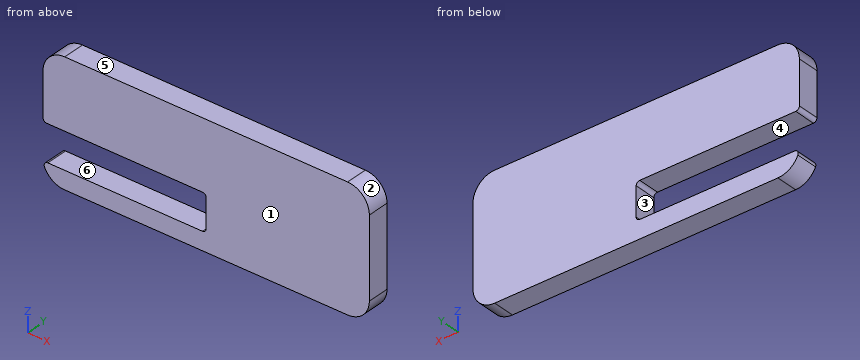
from build123d import *

# Parameters (mm, degrees)
CROQUIS1_W              = 45
CROQUIS1_H              = 17
SALIENTE_EXTRUIR1_DEPTH = 3
CROQUIS2_W              = 22.5
CROQUIS2_H              = 5
CORTAR_EXTRUIR1_DEPTH   = 3
REDONDEO1_R             = 3
REDONDEO4_R             = 0.5


with BuildPart() as part:
    # Croquis1 → Saliente-Extruir1 (new body)
    with BuildSketch(Plane(origin=(0, 0, 0), x_dir=(1, 0, 0), z_dir=(0, 1, 0))):
        with Locations((0, 1.429847209)):
            Rectangle(CROQUIS1_W, CROQUIS1_H)
    extrude(amount=SALIENTE_EXTRUIR1_DEPTH)

    # Croquis2 → Cortar-Extruir1 (cut)
    with BuildSketch(Plane(origin=(0, 3, 0), x_dir=(1, 0, 0), z_dir=(0, 1, 0))):
        with Locations((-11.25, 4.929847209)):
            Rectangle(CROQUIS2_W, CROQUIS2_H)
    extrude(amount=-CORTAR_EXTRUIR1_DEPTH, mode=Mode.SUBTRACT)

    # Redondeo1
    # the kernel refuses this fillet: 3 mm, written as the material it takes off along each edge
    with BuildSketch(Plane(origin=(-22.5, -7.395099729, -9.929847209), x_dir=(1, 0, 0), z_dir=(0, 1, 0))) as redondeo1_piece_1:
        with BuildLine():
            CenterArc((2.958039892, -3), REDONDEO1_R, 90, 80.405931773)
            Line((0, -2.5), (-0.059160798, -2.49))
            ThreePointArc((-0.059160798, -2.49), (-0.06, -1.25), (-0.06, 0))
            Line((-0.06, 0), (0, 0.06))
            Line((0, 0.06), (2.958039892, 0.06))
            Line((2.958039892, 0.06), (2.958039892, 0))
        make_face()
    extrude(amount=17.790199458, mode=Mode.SUBTRACT)
    with BuildSketch(Plane(origin=(22.5, -7.5, -9.929847209), x_dir=(-1, 0, 0), z_dir=(0, 1, 0)), Plane(origin=(22.5, -7.5, 7.070152791), x_dir=(0, 0, -1), z_dir=(0, 1, 0)), Plane(origin=(-22.5, -7.5, 7.070152791), x_dir=(1, 0, 0), z_dir=(0, 1, 0))) as redondeo1_piece_2:
        with BuildLine():
            CenterArc((REDONDEO1_R, REDONDEO1_R), REDONDEO1_R, 180, 90)
            Line((0, REDONDEO1_R), (-REDONDEO1_R * 0.02, REDONDEO1_R))
            Line((-REDONDEO1_R * 0.02, REDONDEO1_R), (-REDONDEO1_R * 0.02, -REDONDEO1_R * 0.02))
            Line((-REDONDEO1_R * 0.02, -REDONDEO1_R * 0.02), (REDONDEO1_R, -REDONDEO1_R * 0.02))
            Line((REDONDEO1_R, -REDONDEO1_R * 0.02), (REDONDEO1_R, 0))
        make_face()
    extrude(amount=18, mode=Mode.SUBTRACT)

    # Redondeo4
    redondeo4_edges = [part.edges().sort_by_distance(p)[0] for p in [
        (-22.5, 1.5, -2.429847209),
        (-22.5, 1.5, -7.429847209),
        (0, 1.5, -7.429847209),
        (0, 1.5, -2.429847209),
    ]]
    fillet(redondeo4_edges, radius=REDONDEO4_R)


solid = part.part
Part model, mm, in its own coordinate system. Face numbers are marked on the shaded views. A direction names the side the tool comes from. Round coordinates to 2 decimals unless told otherwise and drop trailing zeros. Loops run counter-clockwise (first coordinate to the right, second up) from the corner with the lowest first, then second, coordinate; pieces in that order, holes last. Notation, with made-up numbers: (76, 1.25) - (83, 1.25) arc R30 cw to (83, 35.25) - close; hole circle Ø6 at (19.5, 75). An arc over 180 degrees is marked (long way). Answer as a JSON object with one key per item and string values.
Item 1: Pull direction Z, two halves, no side cores. Call the marked faces 1, 2, 3 and 4: pulls with the +Z half, pulls with the -Z half, needs draft (parallel to the pull), parting line crosses it, or undercut.
Output:
{"face 1": "needs draft", "face 2": "pulls with the +Z half", "face 3": "undercut", "face 4": "undercut"}
Item 2: Band-saw the part on A-A on x = -7.5. List the corners of the cut face in (y, z), plus the area to 3 significant figures.
Output:
{"outline": "(0, -9.93) - (3, -9.93) - (3, -7.43) - (0, -7.43) - close; (0, -2.43) - (3, -2.43) - (3, 7.07) - (0, 7.07) - close", "area": "36.0 mm2"}
Item 3: Pin check, flat tip, straight feed: pin 1 (0.9 mm diameter, centred on y = 1, z = -5.5, fed in from -X). Stop position of the tip, or through.
Output:
{"pin 1": "x = 0"}
Item 4: Tool access for the marked faces 5 and 6: list every direction of +Z, -Z, +X, -X, +Y, -Y with a clear straight run to the whole face (end or side of a thin tool).
Output:
{"face 5": "+Z, +X, -X, +Y, -Y", "face 6": "-X, +Y, -Y"}
Item 5: Wall check: L1, parallel to Z at x = -13, y = 1.25; L2, parallel to X at y = 2.65, z = -6; L3, parallel to X at y = 2.4, z = -8.5. Give the ranges that are in metal, low to high.
Output:
{"L1": "-9.93 to -7.43, -2.43 to 7.07", "L2": "0 to 22.5", "L3": "-22.1 to 22.06"}
Item 6: Band-saw the part on B-B on y = 1.95. List the corners of the cut face in (x, z), plus the area to 3 significant figures.
Output:
{"outline": "(-22.5, -1.93) arc R0.5 ccw to (-22, -2.43) - (-0.5, -2.43) arc R0.5 cw to (0, -2.93) - (0, -6.93) arc R0.5 cw to (-0.5, -7.43) - (-21.83, -7.43) arc R0.5 ccw to (-22.29, -8.13) arc R3 ccw to (-19.54, -9.93) - (19.5, -9.93) arc R3 ccw to (22.5, -6.93) - (22.5, 4.07) arc R3 ccw to (19.5, 7.07) - (-19.5, 7.07) arc R3 ccw to (-22.5, 4.07) - close", "area": "645 mm2"}
